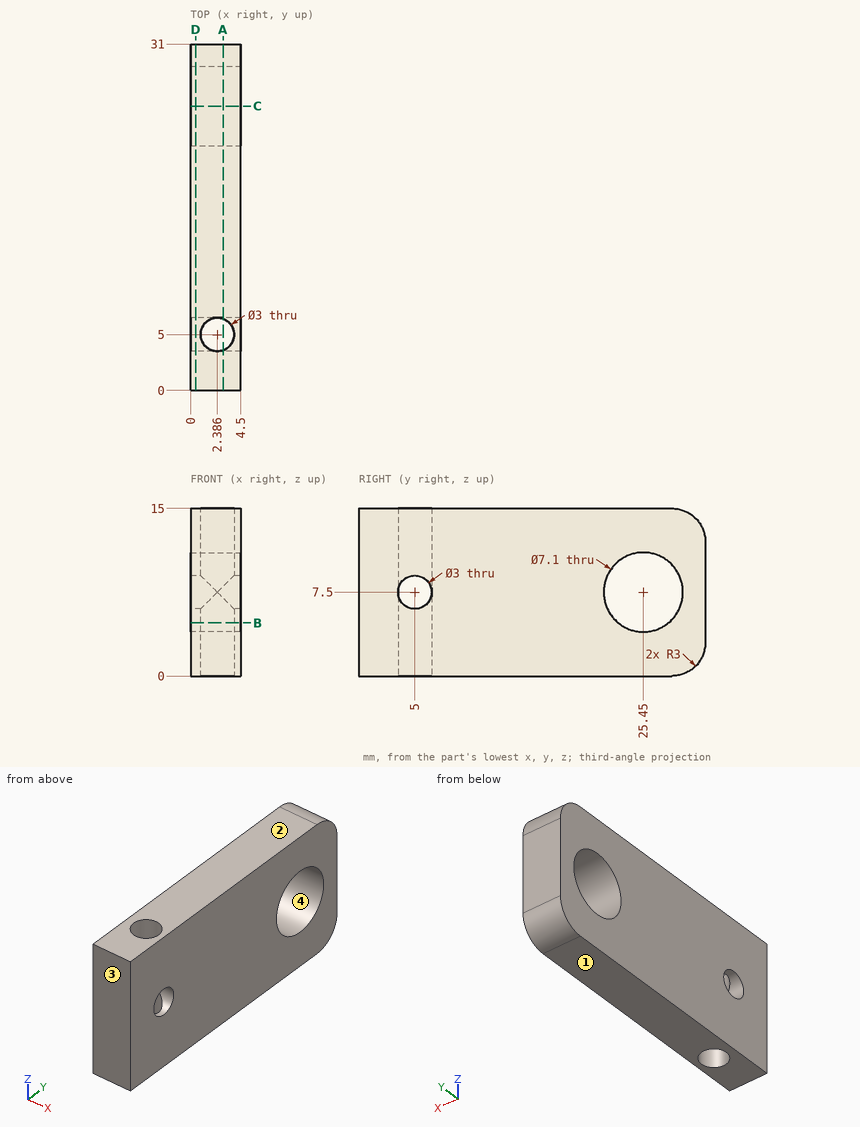
The figure shows three views and two pictorial views of one solid part (mm, origin at its lowest corner). Answer the questions. Give positions to 0.01 mm unless a question says otherwise; leave off trailing zeros. Write each loop counter-clockwise with the first axis right and the second up, starting at its lowest first coordinate (ties: lowest second). Pieces come first, ordered by that corner, then holes. Notation, with made-up numbers: (68.5, 18.25) - (86.5, 18.25) arc R31 ccw to (86.5, 49.25) - close; hole circle Ø1 at (14.5, -40). An arc over 180 degrees is marked (long way). Return JSON: item names as keys, results as strings.
Q1. A cutting plane is placed at A-A, the plane x = 2.9. Determine the outline of the cut face in (y, z), and give its area (3 significant figures).
Reply:
{"outline": "(0, 0) - (3.59, 0) - (3.59, 6.99) arc R1.5 cw to (3.59, 8.01) - (3.59, 15) - (0, 15) - close; (6.41, 0) - (28, 0) arc R3 ccw to (31, 3) - (31, 12) arc R3 ccw to (28, 15) - (6.41, 15) - (6.41, 8.01) arc R1.5 cw to (6.41, 6.99) - close; hole circle Ø7.1 at (25.45, 7.5)", "area": "379 mm²"}
Q2. Consider line 1 along Y through (x, z) = (0.9, 7.5); line 2 along X through (y, z) = (5, 11.25); line 3 along Y through (x, z) = (3.75, 9.5) (1 decimal). Determine where each line is inside the solid, lowest interval first. Write a range as [from, to].
Reply:
{"line 1": "[0, 3.5], [6.5, 21.9], [29, 31]", "line 2": "[0, 0.89], [3.89, 4.5]", "line 3": "[0, 4.4], [5.6, 22.5], [28.4, 31]"}
Q3. A cutting plane is placed at C-C, the plane y = 25.45. Determine the outline of the cut face in (x, z).
Reply:
{"outline": "(0, 0) - (4.5, 0) - (4.5, 3.95) - (0, 3.95) - close; (0, 11.05) - (4.5, 11.05) - (4.5, 15) - (0, 15) - close"}
Q4. A cutting plane is placed at D-D, the plane x = 0.45. Determine the outline of the cut face in (y, z).
Reply:
{"outline": "(0, 0) - (28, 0) arc R3 ccw to (31, 3) - (31, 12) arc R3 ccw to (28, 15) - (0, 15) - close; hole circle Ø3 at (5, 7.5); hole circle Ø7.1 at (25.45, 7.5)"}
Q5. A cutting plane is placed at B-B, the plane z = 4.75. Determine the outline of the cut face in (x, y) (1 decimal), and give its area (3 significant figures).
Reply:
{"outline": "(0, 0) - (4.5, 0) - (4.5, 23.2) - (0, 23.2) - close; (0, 27.7) - (4.5, 27.7) - (4.5, 31) - (0, 31) - close; hole circle Ø3 at (2.4, 5)", "area": "112 mm²"}
Q6. For a pull along Z with two mould halves and no side action, classify the marked faces 1, 2, 3 and 4 as released by +Z, released by -Z, zero draft, split by the parting line, or undercut.
Reply:
{"face 1": "released by -Z", "face 2": "released by +Z", "face 3": "zero draft", "face 4": "undercut"}
